```python
from build123d import *

# Parameters (mm, degrees)
IZIM1_R                     = 10
IZIM1_R_2                   = 9
Y_KSEKLIK_EKSTR_ZYON1_DEPTH = 200
KES_EKSTR_ZYON1_DEPTH       = 200
KES_EKSTR_ZYON1_DEPTH_BACK  = 200
IZIM2_R                     = 2.5
KES_EKSTR_ZYON2_DEPTH       = 200
KES_EKSTR_ZYON2_DEPTH_BACK  = 200
IZIM3_R                     = 2.5


with BuildPart() as part:
    # izim1 → Y_kseklik-Ekstr_zyon1 (new body)
    with BuildSketch(Plane.XY):
        Circle(IZIM1_R)
        Circle(IZIM1_R_2, mode=Mode.SUBTRACT)
    extrude(amount=Y_KSEKLIK_EKSTR_ZYON1_DEPTH)

    # izim2 → Kes-Ekstr_zyon1 (cut, two sides: drawn at the far end of the back side and taken through both)
    with BuildSketch(Plane(origin=(0, 0, 0), x_dir=(1, 0, 0), z_dir=(0, 1, 0)).offset(-KES_EKSTR_ZYON1_DEPTH_BACK)):
        with Locations(Location((0, -10, 0), (0, 0, 270))):
            Circle(IZIM2_R)
        with Locations(Location((0, -60, 0), (0, 0, 270))):
            Circle(IZIM2_R)
    extrude(amount=KES_EKSTR_ZYON1_DEPTH + KES_EKSTR_ZYON1_DEPTH_BACK, mode=Mode.SUBTRACT)

    # izim3 → Kes-Ekstr_zyon2 (cut, two sides: drawn at the far end of the back side and taken through both)
    with BuildSketch(Plane(origin=(0, 0, 0), x_dir=(1, 0, 0), z_dir=(0, 1, 0)).offset(-KES_EKSTR_ZYON2_DEPTH_BACK)):
        with Locations(Location((0, -185, 0), (0, 0, 90))):
            Circle(IZIM3_R)
    extrude(amount=KES_EKSTR_ZYON2_DEPTH + KES_EKSTR_ZYON2_DEPTH_BACK, mode=Mode.SUBTRACT)


solid = part.part
```
Could you check a few things on this model? Use its own coordinates, in mm. Coordinates: 2 decimals unless noted, no trailing zeros. Write each loop counter-clockwise with the first axis right and the second up, starting at its lowest first coordinate (ties: lowest second). Pieces come first, ordered by that corner, then holes. Notation, with made-up numbers: (-5.5, -7.5) -> (14.5, -7.5) arc R11 ccw to (14.5, -1.5) -> close; hole circle Ø4 at (38, 84). An arc over 180 degrees is marked (long way). Return JSON: item names as keys, results as strings.
(1) I'm going to push flat-ended pins straight in: pin 1 (5 mm diameter, centred on x = -7, z = 136, fed in from -Y); pin 2 (5 mm diameter, centred on y = 6.5, z = 110, fed in from +X); pin 3 (4 mm diameter, centred on x = 0, z = 10, fed in from +Y); pin 4 (4 mm diameter, centred on y = -5, z = 77, fed in from -X). Where does each tip first touch, or does it pass through?
Numbers:
{"pin 1": "stops at y = -8.93", "pin 2": "stops at x = 9.17", "pin 3": "passes through", "pin 4": "stops at x = -9.54"}
(2) We'd pull the mould along X, two halves only. Please class faces 1 (the flat face through (-9, 2, 0)), 2 (the cylindrical face through (9.54, 3, 98.6)), 3 (the cylindrical face through (2.11, 9.32, 11.34)): +X half, -X half, draft (parallel to the pull), parting line (faces both ways), or undercut.
Numbers:
{"face 1": "draft", "face 2": "parting line", "face 3": "undercut"}
(3) I need wall thicknesses on L1, parallel to X at y = 0.5, z = 155; L2, parallel to Y at x = -7, z = 172.5; L3, parallel to Y at x = -3.5, z = 134.5. Which ranges of each line are inside material? Lowest first, please.
Numbers:
{"L1": "x = -9.99 to -8.99, 8.99 to 9.99", "L2": "y = -7.14 to -5.66, 5.66 to 7.14", "L3": "y = -9.37 to -8.29, 8.29 to 9.37"}
(4) Imagine slicing it at B-B, the plane z = 185. Please give me the cut outline in (x, y).
Numbers:
{"outline": "(-2.5, -9.68) -> (-2.5, -8.65) arc R9 cw to (-2.5, 8.65) -> (-2.5, 9.68) arc R10 ccw to start; (2.5, -9.68) arc R10 ccw to (2.5, 9.68) -> (2.5, 8.65) arc R9 cw to (2.5, -8.65) -> close"}
(5) Imagine slicing it at A-A, the plane y = 0. Please give me the cut outline in (x, z), then the cut area to 3 significant figures.
Numbers:
{"outline": "(-10, 0) -> (-9, 0) -> (-9, 200) -> (-10, 200) -> close; (9, 0) -> (10, 0) -> (10, 200) -> (9, 200) -> close", "area": "400 mm2"}
(6) Imagine slicing it at C-C, the plane z = 149. Please give me the cut outline in (x, y), then the cut area to 3 significant figures.
Numbers:
{"outline": "circle Ø20 at (0, 0); hole circle Ø18 at (0, 0)", "area": "59.7 mm2"}
